Autodesk Fusion 360 part; units mm, degrees
sketch "Sketch1" plane through (0, 0, 0) normal (0, 0, 1) x (1, 0, 0)
  line L0 (0, 0) -> (55, 0)
  line L1 (55, 0) -> (55, 72)
  line L2 (55, 72) -> (0, 72)
  line L3 (0, 72) -> (0, 0)
  circle A0 centre (27.5, 23.5) radius 3
  line L4 (0, 36) -> (55, 36) construction
  circle A1 centre (27.5, 48.5) radius 3
  dimension "d1" = 55
  dimension "d2" = 72
  dimension "d8" = 6
  dimension "d9" = 25
extrude "Extrude1" add sketch "Sketch1" along normal blind 12
sketch "Sketch2" plane through (0, 0, 12) normal (0, 0, 1) x (-1, 0, 0)
  line L0 (0, -72) -> (0, 0)
  line L1 (0, 0) -> (-55, 0)
  line L2 (-55, 0) -> (-55, -72)
  line L3 (-55, -72) -> (0, -72)
  line L4 (-13.5, 0) -> (-13.5, -72)
  circle A0 centre (-27.5, -23.5) radius 3
  circle A1 centre (-27.5, -48.5) radius 3
  dimension "d5" = 13.5
extrude "Extrude2" cut sketch "Sketch2" against normal blind 2.5 contours L1 L2 L3 L4 | A0 | A1
fillet "Fillet1" radius 3 4 edges at (0, 0, 6) (55, 0, 4.75) (55, 72, 4.75) (0, 72, 6)
The listing builds one solid part. Answer for the finished solid, in the listing's coordinates (mm). A direction names the side the tool comes from. Round coordinates to 2 decimals unless told otherwise and drop trailing zeros. Write each loop counter-clockwise with the first axis right and the second up, starting at its lowest first coordinate (ties: lowest second). Pieces come first, ordered by that corner, then holes. Notation, with made-up numbers: (-19.5, -31) -> (0.5, -31) arc R29 ccw to (0.5, -11) -> close; hole circle Ø4 at (67.5, 28). An arc over 180 degrees is marked (long way). Answer as a JSON object with one key per item and string values. Group by question number.
Q1. Section B-B (z = 7) is taken. Write down the section's boundary in (x, y).
Q2. Section D-D (z = 10.25) is taken. Write down the section's boundary in (x, y).
Q3. Each of these flat-tipped pins is pushed along its axis until it touches: pin 1 Ø2 at (y, z) = (39, 11) entering from +X; pin 2 Ø1 at (x, y) = (44.5, 11.5) entering from +Z. Where does it stop, or does it pass through?
Q4. Straight lines are drawn through the part: line 1 along Y through (x, z) = (27.5, 3.25); line 2 along X through (y, z) = (23.5, 4); line 3 along Z through (x, y) = (27, 44.5). For each, find the intervals that lie inside material, in ascending order.
Q5. Section A-A (y = 23.5) is taken. Write down the section's boundary in (x, z), plus the area to 3 significant figures.
Q6. Section C-C (x = 28.5) is taken. Write down the section's boundary in (y, z).
Q7. Which of the six approach directions +Z, -Z, +X, -X, +Y, -Y give full straight-line access (tool end or side, diameter ignored) to faces 1 (the face through (13.5, 35, 11)), 2 (the face through (0.86, 0.9, 6.08))?
Check values:
{
 "1": {"outline": "(0, 3) arc R3 ccw to (3, 0) -> (52, 0) arc R3 ccw to (55, 3) -> (55, 69) arc R3 ccw to (52, 72) -> (3, 72) arc R3 ccw to (0, 69) -> close; hole circle Ø6 at (27.5, 23.5); hole circle Ø6 at (27.5, 48.5)"},
 "2": {"outline": "(0, 3) arc R3 ccw to (3, 0) -> (13.5, 0) -> (13.5, 72) -> (3, 72) arc R3 ccw to (0, 69) -> close"},
 "3": {"pin 1": "x = 13.5", "pin 2": "z = 9.5"},
 "4": {"line 1": "0 to 20.5, 26.5 to 45.5, 51.5 to 72", "line 2": "0 to 24.5, 30.5 to 55", "line 3": "0 to 9.5"},
 "5": {"outline": "(0, 0) -> (24.5, 0) -> (24.5, 9.5) -> (13.5, 9.5) -> (13.5, 12) -> (0, 12) -> close; (30.5, 0) -> (55, 0) -> (55, 9.5) -> (30.5, 9.5) -> close", "area": "499 mm^2"},
 "6": {"outline": "(0, 0) -> (20.67, 0) -> (20.67, 9.5) -> (0, 9.5) -> close; (26.33, 0) -> (45.67, 0) -> (45.67, 9.5) -> (26.33, 9.5) -> close; (51.33, 0) -> (72, 0) -> (72, 9.5) -> (51.33, 9.5) -> close"},
 "7": {"face 1": "+Z, +X, +Y, -Y", "face 2": "+Z, -Z, -X, -Y"}
}
